```python
from build123d import *

# Parameters (mm, degrees)
F0_R     = 3
F1_DEPTH = 5
F2_R     = 1


# Not quite as in the source:
# - a feature names something its author has since deleted; it is built from what else it names


with BuildPart() as f1:
    # F0 (on Front) → F1 (new body)
    with BuildSketch(Plane.XZ):
        Polygon((-3.4352341017, 5.95), (-6.8704682034, 0), (-3.4352341017, -5.95), (3.4352341017, -5.95), (6.8704682034, 0), (3.4352341017, 5.95), align=None)
        Circle(F0_R, mode=Mode.SUBTRACT)
    extrude(amount=F1_DEPTH)

    # F2
    f2_edges = [f1.edges().sort_by_distance(p)[0] for p in [
        (-3.435234, -2.5, 5.95),
        (-6.870468, -2.5, 0),
        (-3.435234, -2.5, -5.95),
        (3.435234, -2.5, 5.95),
        (6.870468, -2.5, 0),
        (3.435234, -2.5, -5.95),
        (5.152851, -5, -2.975),
        (5.152851, 0, -2.975),
        (5.152851, 0, 2.975),
        (5.152851, -5, 2.975),
        (0, -5, -5.95),
        (0, 0, -5.95),
        (-5.152851, 0, -2.975),
        (-5.152851, -5, -2.975),
        (-5.152851, -5, 2.975),
        (0, -5, 5.95),
        (0, 0, 5.95),
        (-5.152851, 0, 2.975),
    ]]
    fillet(f2_edges, radius=F2_R)


solid = f1.part
```
Input: part model. Units: mm. Frame: model coordinates. Coordinates: 2 decimals unless noted, no trailing zeros. Order: outer loops, then holes, each group sorted by start corner. A loop starts at its lowest first (then second) coordinate and runs counter-clockwise, first axis right, second up. Notation, with made-up numbers: (31, 73) - (45, 73) arc R8 ccw to (45, 87) - close; hole circle Ø5 at (25, -12.75). An arc over 180 degrees is marked (long way). Return JSON: item names as keys, results as strings.
Q1. Cut plane B-B (y = -2.4). Return loops of the section in (x, z), then the cut area to 3 significant figures.
The answers:
{"outline": "(-6.58, -0.5) - (-3.72, -5.45) arc R1 ccw to (-2.86, -5.95) - (2.86, -5.95) arc R1 ccw to (3.72, -5.45) - (6.58, -0.5) arc R1 ccw to (6.58, 0.5) - (3.72, 5.45) arc R1 ccw to (2.86, 5.95) - (-2.86, 5.95) arc R1 ccw to (-3.72, 5.45) - (-6.58, 0.5) arc R1 ccw to start; hole circle Ø6 at (0, 0)", "area": "94.0 mm2"}
Q2. Cut plane A-A (x = 0). Return loops of the section in (y, z), then the cut area to 3 significant figures.
The answers:
{"outline": "(-5, -4.95) arc R1 ccw to (-4, -5.95) - (-1, -5.95) arc R1 ccw to (0, -4.95) - (0, -3) - (-5, -3) - close; (-5, 3) - (0, 3) - (0, 4.95) arc R1 ccw to (-1, 5.95) - (-4, 5.95) arc R1 ccw to (-5, 4.95) - close", "area": "28.6 mm2"}
Q3. First-contact query: pin 1 (2 mm diameter, centred on x = -1, z = 3.5, fed in from +Y). Flat tip, straight axial feed; report the tip coordinate or a pass-through.
The answers:
{"pin 1": "stops at y = 0"}
Q4. Draft query along Z for faces 1 (the flat face through (-5.133, -2.479, 3.01)), 2 (the cylindrical face through (4.926, -0.301, -2.798)), 3 (the cylindrical face through (-3, -2, 0)). Return one class per face: +Z half, -Z half, draft (parallel to the pull), parting line (faces both ways), or undercut.
The answers:
{"face 1": "+Z half", "face 2": "-Z half", "face 3": "undercut"}
Q5. Cut plane C-C (y = -4.5). Return loops of the section in (x, z), then the cut area to 3 significant figures.
The answers:
{"outline": "(-6.47, -0.43) - (-3.61, -5.38) arc R0.87 ccw to (-2.86, -5.82) - (2.86, -5.82) arc R0.87 ccw to (3.61, -5.38) - (6.47, -0.43) arc R0.87 ccw to (6.47, 0.43) - (3.61, 5.38) arc R0.87 ccw to (2.86, 5.82) - (-2.86, 5.82) arc R0.87 ccw to (-3.61, 5.38) - (-6.47, 0.43) arc R0.87 ccw to start; hole circle Ø6 at (0, 0)", "area": "88.7 mm2"}
Q6. Ray query, probe 1 along Z at (x, y) = (0, -1.55); probe 2 along X at (y, z) = (-1.05, -2.25); probe 3 along Z at (x, y) = (-3.5, -1). Return the intervals inside material, ascending.
The answers:
{"probe 1": "z = -5.95 to -3, 3 to 5.95", "probe 2": "x = -5.57 to -1.98, 1.98 to 5.57", "probe 3": "z = -5.72 to 5.72"}
